Autodesk Inventor part; units mm, degrees
ref_plane "YZ Plane" through (0, 0, 0) normal (1, 0, 0) x (0, 1, 0)
ref_plane "XZ Plane" through (0, 0, 0) normal (0, 1, 0) x (-1, 0, 0)
ref_plane "XY Plane" through (0, 0, 0) normal (0, 0, 1) x (1, 0, 0)
sketch "Sketch1" plane through (0, 0, 0) normal (0, 1, 0) x (-1, 0, 0)
  line L0 (3.6662, -6.35) -> (-3.6662, -6.35)
  line L1 (-3.6662, -6.35) -> (-7.3323, 0)
  line L2 (-7.3323, 0) -> (-3.6662, 6.35)
  line L3 (-3.6662, 6.35) -> (3.6662, 6.35)
  line L4 (3.6662, 6.35) -> (7.3323, 0)
  line L5 (7.3323, 0) -> (3.6662, -6.35)
  point P0 (0, 0)
  point P1 (0, 0)
  dimension "d0" = 12.7
extrude "Extrusion1" add sketch "Sketch1" against normal blind 42.8625
sketch "Sketch2" plane through (0, 0, 0) normal (0, 1, 0) x (1, 0, 0)
  circle A0 centre (0, 0) radius 4.7625
  dimension "d3" = 9.525
extrude "Extrusion2" add sketch "Sketch2" along normal blind 52.3875
sketch "Sketch3" plane through (0, -42.8625, 0) normal (0, -1, 0) x (1, 0, 0)
  circle A0 centre (0, 0) radius 4.7625
  circle A1 centre (0, 0) radius 1.905
  dimension "d7" = 3.81
extrude "Extrusion3" cut sketch "Sketch3" against normal blind 25.4 contours A1
properties part number "Roller drive shaft" material "Aluminum 6061"
The listing builds one solid part. Answer for the finished solid, in the listing's coordinates (mm). A direction names the side the tool comes from. Give positions to 0.01 mm unless a question says otherwise; leave off trailing zeros. Loops run counter-clockwise (first coordinate to the right, second up) from the corner with the lowest first, then second, coordinate; pieces in that order, holes last.
Item 1: Find the intervals of material crossed by line 1 along Z through (x, y) = (0, -32.25) (3 decimals); line 2 along Z through (x, y) = (-0.25, 18); line 3 along Y through (x, z) = (-0.5, 0), in increasing order.
Derived:
line 1: z = -6.35 to -1.905, 1.905 to 6.35
line 2: z = -4.76 to 4.76
line 3: y = -17.46 to 52.39
Item 2: A cutting plane is placed at C-C (y = -13). Give the vertices of the cut face in (x, z).
Derived:
outline: (-7.33, 0) - (-3.67, -6.35) - (3.67, -6.35) - (7.33, 0) - (3.67, 6.35) - (-3.67, 6.35) - close
Item 3: Each of these flat-tipped pins is pushed along its axis until it touches: pin 1 Ø1.5 at (x, z) = (3.5, -4.5) entering from +Y; pin 2 Ø1 at (x, y) = (-5, -23.5) entering from -Z; pin 3 Ø2 at (y, z) = (34, 5) entering from +X; pin 4 Ø4 at (x, z) = (0.5, -1) entering from -Y. Where does it stop, or does it pass through?
Derived:
pin 1: stops at y = 0
pin 2: stops at z = -4.91
pin 3: stops at x = 2.58
pin 4: stops at y = -42.86
Item 4: A cutting plane is placed at B-B (z = 3.5). Give the vertices of the cut face in (x, y).
Derived:
outline: (-5.31, -42.86) - (5.31, -42.86) - (5.31, 0) - (3.23, 0) - (3.23, 52.39) - (-3.23, 52.39) - (-3.23, 0) - (-5.31, 0) - close
Item 5: A cutting plane is placed at D-D (y = 13). Give the vertices of the cut face in (x, z) (1 decimal), then the cut area to 3 significant figures.
Derived:
outline: circle Ø9.5 at (0, 0)
area: 71.3 mm2
Item 6: Determine the mould class of faces 3 (the flat face through (0, -21, 6.35)), 4 (the flat face through (0, -17.462, 0)), 5 (the cylindrical face through (-0.41, -30.34, -1.86)), 6 (the flat face through (-5.474, -21.131, 3.219)) for opening direction X: +X half, -X half, draft (parallel to the pull), parting line (faces both ways), or undercut.
Derived:
face 3: draft
face 4: undercut
face 5: undercut
face 6: -X half
Item 7: A tool of negligible diameter and unlimited length cuts with its end or side. For faces 1 (the flat face through (-5.525, -21.131, -3.131)), 2 (the flat face through (-5, 0, 0)), from which of +Z, -Z, +X, -X, +Y, -Y can it reach the whole face along a straight path? Write none if from no direction.
Derived:
face 1: -Z, -X, +Y, -Y
face 2: +Y
